```python
from build123d import *
from build123d.topology import SkipClean

# Parameters (mm, degrees)
CROQUIS1_R                   = 27.65
SALIENTE_EXTRUIR1_DEPTH      = 21.9
SALIENTE_EXTRUIR2_DEPTH      = 8.8
SALIENTE_EXTRUIR2_DEPTH_BACK = 34
CROQUIS2_R                   = 2
SALIENTE_EXTRUIR3_START      = 1.7
CROQUIS3_R                   = 2.25
CROQUIS3_R_2                 = 2
SALIENTE_EXTRUIR3_DEPTH      = 1.7
CROQUIS4_R                   = 5.55
SALIENTE_EXTRUIR4_DEPTH      = 2


with BuildPart() as part:
    # Croquis1 → Saliente-Extruir1 (new body)
    with BuildSketch(Plane.XY):
        Circle(CROQUIS1_R)
    extrude(amount=SALIENTE_EXTRUIR1_DEPTH)

    # Croquis2 → Saliente-Extruir2 (add, two sides: drawn at the far end of the back side and taken through both)
    with BuildSketch(Plane.XY.offset(21.9).offset(-SALIENTE_EXTRUIR2_DEPTH_BACK)):
        Circle(CROQUIS2_R)
    extrude(amount=SALIENTE_EXTRUIR2_DEPTH + SALIENTE_EXTRUIR2_DEPTH_BACK)

    # Croquis3 → Saliente-Extruir3 (add)
    with SkipClean():  # the faces are left unmerged after this step: merging them gives an invalid solid
        with BuildSketch(Plane(origin=(0, 0, 0), x_dir=(-1, 0, 0), z_dir=(0, 0, -1)).offset(SALIENTE_EXTRUIR3_START)):
            with BuildLine():
                Line((27.194162977, -5), (33.5, -5))
                ThreePointArc((33.5, -5), (38.159388464, -1.813863043), (36.880597015, 3.683960345))
                Line((36.880597015, 3.683960345), (18.694701493, 20.372300707))
                ThreePointArc((18.694701493, 20.372300707), (-0.0770274, 27.649892708), (-18.80791724, 20.267825466))
                Line((-18.80791724, 20.267825466), (-35.955174002, 4.355699785))
                ThreePointArc((-35.955174002, 4.355699785), (-38.336243321, -1.269153473), (-33.5, -5))
                Line((-33.5, -5), (-27.194162977, -5))
                ThreePointArc((-27.194162977, -5), (0, -27.65), (27.194162977, -5))
            make_face()
            with Locations((33.5, 0)):
                Circle(CROQUIS3_R, mode=Mode.SUBTRACT)
            with Locations(Location((0, 0, 0), (0, 0, 180))):
                Circle(CROQUIS3_R_2, mode=Mode.SUBTRACT)
            with Locations((-33.5, 0)):
                Circle(CROQUIS3_R, mode=Mode.SUBTRACT)
        extrude(amount=-SALIENTE_EXTRUIR3_DEPTH)

    # Croquis4 → Saliente-Extruir4 (add)
    with SkipClean():  # the faces are left unmerged after this step: merging them gives an invalid solid
        with BuildSketch(Plane(origin=(0, 0, -1.7), x_dir=(-1, 0, 0), z_dir=(0, 0, -1))):
            Circle(CROQUIS4_R)
        extrude(amount=SALIENTE_EXTRUIR4_DEPTH)


solid = part.part
```
Here's how the part is built. I have some questions about the finished solid (model axes, mm). A direction names the side the tool comes from. Round coordinates to 2 decimals unless told otherwise and drop trailing zeros. Order: outer loops, then holes, each group sorted by start corner. A loop starts at its lowest first (then second) coordinate and runs counter-clockwise, first axis right, second up. Notation, with made-up numbers: M 16.25,-6 L 59.25,-6 A17 ccw 59.25,7 Z; hole C -6,78.5 d7. An arc over 180 degrees is marked long. Use CSV: the item, a comma, the result in double quotes.
1) On a 3-axis mill with a long thin cutter (end or side, diameter ignored), from which of +Z, -Z, +X, -X, +Y, -Y can I reach the whole of each face in a straight line? I mean faces 1 (the cylindrical face through (0, -2, -8)), 2 (the flat face through (-30, -5, -1)), 3 (the flat face through (30, -5, -1)), 4 (the cylindrical face through (-38.13, -1.89, -0.86)), 5 (the cylindrical face through (0, -2, 26)). Say none if no direction works.
Taken from the geometry:
face 1,"-Z"
face 2,"+Z, -Z, -X, -Y"
face 3,"+Z, -Z, +X, -Y"
face 4,"+Z, -Z, -X"
face 5,"+Z"
2) I want a section at B-B (y = 10.5). List the corners of the cut face in (x, z) for me, then the cut area to 3 significant figures.
Taken from the geometry:
outline,"M -29.45,-1.7 L 29.33,-1.7 L 29.33,0 L 25.58,0 L 25.58,21.9 L -25.58,21.9 L -25.58,0 L -29.45,0 Z"
area,"1,220 mm^2"
3) I need wall thicknesses on line 1 along Z through (x, y) = (-4, -3); line 2 along Z through (x, y) = (17.5, -8); line 3 along Y through (x, z) = (5, 11). Which ranges of each line are inside material? Lowest first, please. Write a range as [from, to].
Taken from the geometry:
line 1,"[-3.7, 21.9]"
line 2,"[-1.7, 21.9]"
line 3,"[-27.19, 27.19]"
4) If we mould it in two halves opening along X, with no side actions, what happens to faces 6 (the cylindrical face through (-35.58, -0.86, -0.86)), 7 (the cylindrical face through (-2.98, 4.68, -2.69)), 8 (the flat face through (1, 7, -1.7))? For each: pulls with the +X half, pulls with the -X half, needs draft (parallel to the pull), parting line crosses it, or undercut.
Taken from the geometry:
face 6,"undercut"
face 7,"parting line crosses it"
face 8,"needs draft"
5) I'm going to push flat-ended pins straight in: P1, Ø0.8, axis at x = 31, z = -1, coming from the -Y side; P2, Ø3, axis at x = -17.5, z = -3, coming from the +Y side; P3, Ø5, axis at x = -30.5, z = 23.5, coming from the -Y side; P4, Ø5, axis at x = 7.5, y = -16.5, coming from the +Z side. Where does each tip first touch, or does it pass through?
Taken from the geometry:
P1,"y = -5"
P2,"y = 22"
P3,"through"
P4,"z = 21.9"
6) I want a section at C-C (z = 20). List the corners of the cut face in (x, y) for me.
Taken from the geometry:
outline,"C 0,0 d55.3"
7) I want a section at A-A (x = 0). List the corners of the cut face in (y, z) for me, then the cut area to 3 significant figures.
Taken from the geometry:
outline,"M -27.65,-1.7 L -5.55,-1.7 L -5.55,-3.7 L -2,-3.7 L -2,-12.1 L 2,-12.1 L 2,-3.7 L 5.55,-3.7 L 5.55,-1.7 L 27.65,-1.7 L 27.65,21.9 L 2,21.9 L 2,30.7 L -2,30.7 L -2,21.9 L -27.65,21.9 Z"
area,"1,400 mm^2"
8) I want a section at D-D (x = 23.5). List the corners of the cut face in (y, z) for me, then the cut area to 3 significant figures.
Taken from the geometry:
outline,"M -14.57,-1.7 L 15.91,-1.7 L 15.91,0 L 14.57,0 L 14.57,21.9 L -14.57,21.9 Z"
area,"690 mm^2"
